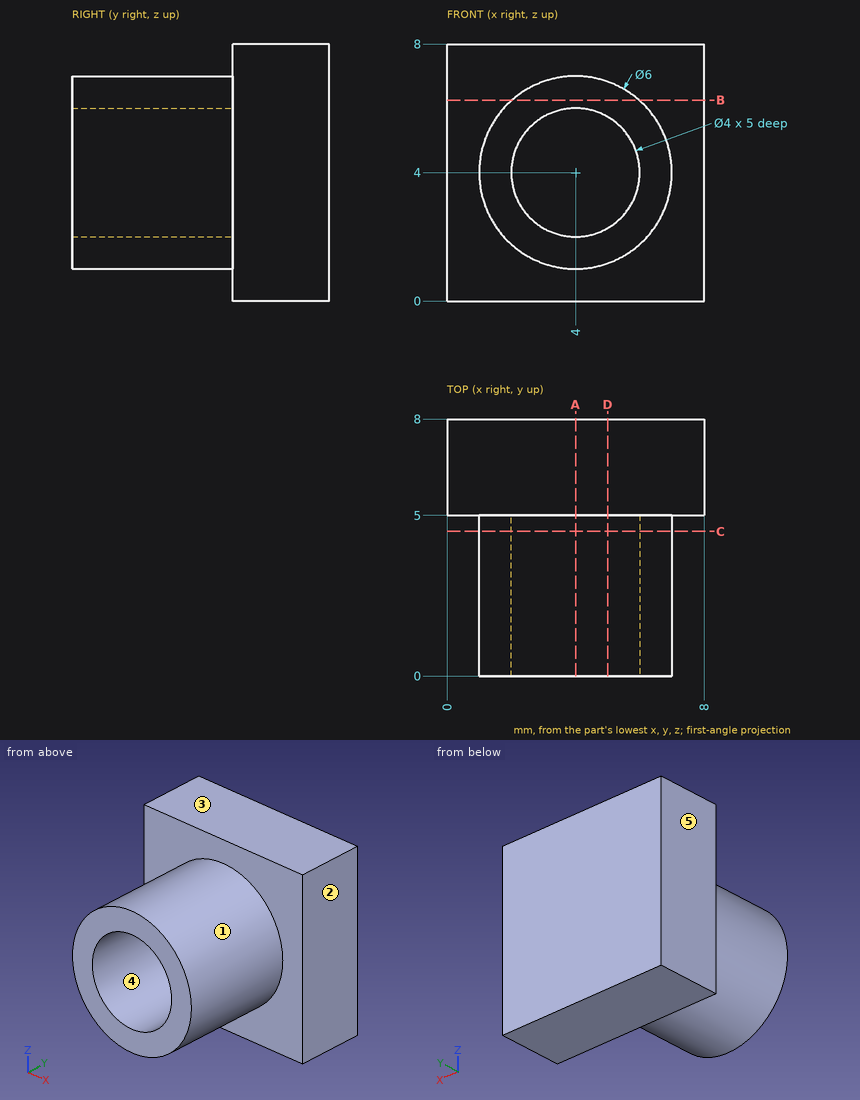
Here's the drawing with two shaded views (mm, measured from the low corner). I have some questions. A direction names the side the tool comes from. Coordinates: 2 decimals unless noted, no trailing zeros. Write each loop counter-clockwise with the first axis right and the second up, starting at its lowest first coordinate (ties: lowest second). Pieces come first, ordered by that corner, then holes. Notation, with made-up numbers: M 59,-18.5 L 116,-18.5 A26 cw 116,-0.5 Z; hole C 77.25,16 d3. An arc over 180 degrees is marked long. Answer as CSV lines item,"result". Start each with the question number.
1) I want a section at D-D, the plane x = 5. Please give me the cut outline in (y, z).
2) I want a section at B-B, the plane z = 6.25. Please give me the cut outline in (x, y), and give its area (3 significant figures).
3) I want a section at C-C, the plane y = 4.5. Please give me the cut outline in (x, z).
4) For P1, Ø1.2, axis at x = 3, z = 4, coming from the -Y side; P2, Ø1.5, axis at y = 6.5, z = 3, coming from the -X side, each with a flat end and sliding along its axis, tell me the tip position at first contact or that it passes through.
5) I want a section at A-A, the plane x = 4. Please give me the cut outline in (y, z), and give its area (3 significant figures).
6) We'd pull the mould along Z, two halves only. Please class the marked faces 3, 4 and 5: +Z half, -Z half, draft (parallel to the pull), parting line (faces both ways), or undercut.
7) For the marked faces 1 and 2, which set-ups out of +Z, -Z, +X, -X, +Y, -Y let a thin tool reach every point of the face, with its end or its side?
8) Please list where these lines run through material, in increasing order: line 1 (Z direction, x = 4, y = 2.95); line 2 (Y direction, x = 3.25, z = 3.25); line 3 (Z direction, x = 5.75, y = 0.5). Write a range as from..to.
Data:
1,outline,"M 0,1.17 L 5,1.17 L 5,0 L 8,0 L 8,8 L 5,8 L 5,6.83 L 0,6.83 L 0,5.73 L 5,5.73 L 5,2.27 L 0,2.27 Z"
2,outline,"M 0,5 L 2.02,5 L 2.02,0 L 5.98,0 L 5.98,5 L 8,5 L 8,8 L 0,8 Z"
2,area,"43.8 mm^2"
3,outline,"C 4,4 d6; hole C 4,4 d4"
4,P1,"stops at y = 5"
4,P2,"stops at x = 0"
5,outline,"M 0,1 L 5,1 L 5,0 L 8,0 L 8,8 L 5,8 L 5,7 L 0,7 L 0,6 L 5,6 L 5,2 L 0,2 Z"
5,area,"34.0 mm^2"
6,face 3,"+Z half"
6,face 4,"undercut"
6,face 5,"draft"
7,face 1,"-Y"
7,face 2,"+Z, -Z, +X, +Y, -Y"
8,line 1,"z = 1..2, 6..7"
8,line 2,"y = 5..8"
8,line 3,"z = 1.56..3.03, 4.97..6.44"
